Autodesk Inventor part; units mm, degrees
ref_plane "YZ Plane" through (0, 0, 0) normal (1, 0, 0) x (0, 1, 0)
ref_plane "XZ Plane" through (0, 0, 0) normal (0, 1, 0) x (-1, 0, 0)
ref_plane "XY Plane" through (0, 0, 0) normal (0, 0, 1) x (1, 0, 0)
sketch "Sketch2" plane through (0, -7.5, 2.5) normal (1, 0, 0) x (0, 1, 0)
  line L0 (0, 0) -> (12.5, 0)
  line L1 (12.5, 0) -> (12.5, -5)
  line L2 (12.5, -5) -> (0, -5)
  line L3 (0, 0) -> (0, 5)
  line L4 (0, 5) -> (15, 5)
  line L5 (15, 5) -> (15, -10)
  line L6 (15, -10) -> (0, -10)
  line L7 (0, -10) -> (0, -5)
  dimension "d11" = 12.5
  dimension "d10" = 5
  dimension "d9" = 15
  dimension "d8" = 15
  dimension "d12" = 5
extrude "Extrusion2" add sketch "Sketch2" along normal blind 22
sketch "Sketch4" plane through (0, -7.5, -7.5) normal (0, 0, -1) x (-1, 0, 0)
  line L0 (0, 0) -> (0, 15)
  line L1 (0, 15) -> (-22, 15)
  line L2 (-22, 0) -> (-22, 15)
  line L3 (0, 0) -> (-22, 0)
  line L4 (5.5, 15) -> (-31.5, 15)
  line L5 (-31.5, 37) -> (-31.5, 34.5)
  line L6 (5.5, 15) -> (5.5, 37)
  line L7 (5.5, 37) -> (3, 37)
  line L8 (3, 34.5) -> (3, 17.5)
  line L9 (3, 17.5) -> (-31.5, 17.5)
  line L10 (-31.5, 17.5) -> (-31.5, 15)
  line L11 (3, 37) -> (-31.5, 37)
  line L12 (3, 34.5) -> (-31.5, 34.5)
  point P0 (0, 7.5)
  dimension "d29" = 5.5
  dimension "d32" = 19.5
  dimension "d33" = 2.5
  dimension "d34" = 2.5
  dimension "d35" = 22
  dimension "d38" = 15
  dimension "d58" = 2.5
  dimension "d65" = 37
  dimension "d66" = 34.5
  dimension "d67" = 2.5
extrude "Extrusion4" add sketch "Sketch4" against normal blind 20 and the other way blind 5 contours L1 L4 L10 L9 L8 L12 L5 L11 L7 L6
sketch "Sketch9" plane through (0, -7.5, 12.5) normal (0, 0, 1) x (1, 0, 0)
  line L0 (-5.5, 37) -> (31.5, 37)
  line L1 (-5.5, 37) -> (-5.5, 15)
  line L2 (31.5, 37) -> (-5.5, 37)
  line L3 (-5.5, 37) -> (-5.5, 15)
  line L4 (-5.5, 15) -> (31.5, 15)
  line L5 (31.5, 15) -> (31.5, 37)
  point P0 (0, 7.5)
extrude "Extrusion9" add sketch "Sketch9" along normal blind 2.5
sketch "Sketch10" plane through (31.5, 7.5, -12.5) normal (1, 0, 0) x (0, 0, -1)
  line L0 (-27.5, 22) -> (-27.5, 0)
  line L1 (0, 0) -> (-27.5, 0)
  line L2 (-27.5, 11) -> (0, 11)
  line L3 (0, 11) -> (0, 0)
  line L4 (0, 0) -> (-27.5, 0)
  line L5 (-27.5, 0) -> (-27.5, 11)
  point P0 (-12.5, -7.5)
extrude "Extrusion10" cut sketch "Sketch10" against normal blind 7.5
properties part number "battery-holder-two"
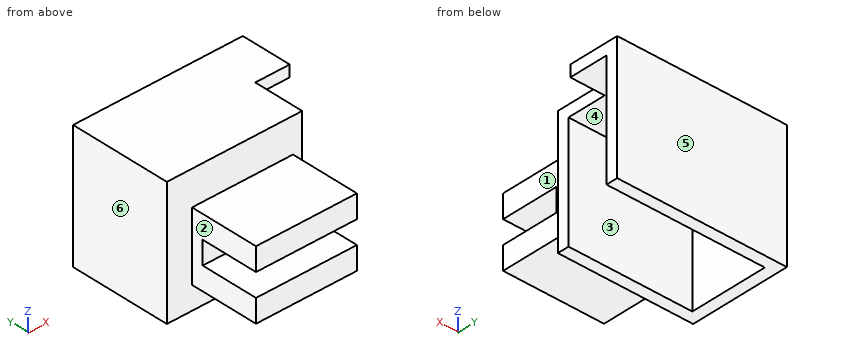
Verification items for the finished model (mm, model axes). Face numbers are marked on the shaded views. A direction names the side the tool comes from. Round coordinates to 2 decimals unless told otherwise and drop trailing zeros. Order: outer loops, then holes, each group sorted by start corner. A loop starts at its lowest first (then second) coordinate and runs counter-clockwise, first axis right, second up. Notation, with made-up numbers: (18, 32) - (73, 32) arc R31 ccw to (73, 61) - close; hole circle Ø7 at (50, 22.5). An arc over 180 degrees is marked (long way). Use CSV: the item, a comma, the result in double quotes.
(1) Section check D-D on z = 10.5. Record the boundary of the cut face in (x, y).
Entries:
outline,"(-5.5, 7.5) - (24, 7.5) - (24, 10) - (-3, 10) - (-3, 27) - (31.5, 27) - (31.5, 29.5) - (-5.5, 29.5) - close"
(2) Section check A-A on y = 2.5. Record the boundary of the cut face in (x, z).
Entries:
outline,"(0, -7.5) - (22, -7.5) - (22, -2.5) - (0, -2.5) - close; (0, 2.5) - (22, 2.5) - (22, 7.5) - (0, 7.5) - close"
(3) Mould release check, pull along Y, two halves, no side actions. Record for the marked faces 4, 5 and 6: released by +Y, released by -Y, zero draft, split by the parting line, or undercut.
Entries:
face 4,"undercut"
face 5,"released by +Y"
face 6,"zero draft"
(4) Section check C-C on x = 27. Record the boundary of the cut face in (y, z), and give its area (3 significant figures).
Entries:
outline,"(18.5, 12.5) - (27, 12.5) - (27, -12.5) - (29.5, -12.5) - (29.5, 15) - (18.5, 15) - close"
area,"90.0 mm^2"
(5) Thickness scan on probe 1 along Y at (x, z) = (12.5, 2); probe 2 along Z at (x, y) = (16, 1.5); probe 3 along Y at (x, z) = (-0.5, 7.5). Record the ranges inside material, lowest first. Write a range as from..to.
Entries:
probe 1,"5..10, 27..29.5"
probe 2,"-7.5..-2.5, 2.5..7.5"
probe 3,"7.5..10, 27..29.5"
(6) Gauge pin test, flat ends, axial feed: pin 1 Ø4.5 at (x, y) = (9.5, -1) entering from -Z; pin 2 Ø7.5 at (y, z) = (0, -3) entering from +X; pin 3 Ø5 at (y, z) = (17.5, 2) entering from +X; pin 4 Ø13.5 at (x, y) = (14, 16) entering from -Z. Record the tip position at first contact, or that the pin passes through.
Entries:
pin 1,"z = -7.5"
pin 2,"x = 22"
pin 3,"x = -3"
pin 4,"z = -12.5"
(7) Section check B-B on z = -3.75. Record the boundary of the cut face in (x, y), and give its area (3 significant figures).
Entries:
outline,"(-5.5, 7.5) - (0, 7.5) - (0, -7.5) - (22, -7.5) - (22, 7.5) - (24, 7.5) - (24, 10) - (-3, 10) - (-3, 27) - (31.5, 27) - (31.5, 29.5) - (-5.5, 29.5) - close"
area,"539 mm^2"
(8) Access from +Z, -Z, +X, -X, +Y, -Y to the whole of each face (thin tool, end or side, straight path). Record for the marked faces 1, 2 and 3.
Entries:
face 1,"+Z, -Z, +X, -Y"
face 2,"+Z, -Z, -X, -Y"
face 3,"-Z, +X"
